Build history of the part. All positions in model axes, mm. Face numbers are marked on the shaded views. A direction names the side the tool comes from. Give positions to 0.01 mm unless a question says otherwise; leave off trailing zeros. Order: outer loops, then holes, each group sorted by start corner. A loop starts at its lowest first (then second) coordinate and runs counter-clockwise, first axis right, second up. Notation, with made-up numbers: (65, 81) - (86, 81) arc R16 cw to (86, 100) - close; hole circle Ø10 at (22, 82.5). An arc over 180 degrees is marked (long way). Answer in a Markdown table with one row per item.
```python
from build123d import *

# Parameters (mm, degrees)
SPUR_START          = 60.68508869
SPUR_GEAR_AI_DEPTH  = 13.97
SKETCH1_R           = 8.73125
BOSS_EXTRUDE1_DEPTH = 0.381
BOSS_EXTRUDE2_START = 0.381
SKETCH2_R           = 8.73125
BOSS_EXTRUDE2_DEPTH = 0.381


# Read off the part's stored shape, not the designer's step: spur gear_ai
with BuildPart() as part:
    # spur gear_ai outline → spur gear_ai (new body)
    with BuildSketch(Plane.YZ.offset(SPUR_START)):
        with BuildLine():
            ThreePointArc((-11.323917399, -24.217086363), (-11.097675416, -23.865456059), (-10.883753605, -23.506197427))
            ThreePointArc((-10.883753605, -23.506197427), (-11.804950291, -22.339121223), (-13.067398654, -21.553695012))
            ThreePointArc((-13.067398654, -21.553695012), (-12.757964709, -20.844772424), (-12.509041094, -20.112408009))
            ThreePointArc((-12.509041094, -20.112408009), (-11.04694228, -20.382476998), (-9.57991556, -20.14060347))
            ThreePointArc((-9.57991556, -20.14060347), (-9.495974711, -19.730989946), (-9.42627775, -19.318713778))
            ThreePointArc((-9.42627775, -19.318713778), (-10.70686463, -18.563222253), (-12.167791342, -18.286883074))
            ThreePointArc((-12.167791342, -18.286883074), (-12.135345159, -17.514052013), (-12.167791342, -16.741220953))
            ThreePointArc((-12.167791342, -16.741220953), (-10.70686463, -16.464881774), (-9.42627775, -15.709390249))
            ThreePointArc((-9.42627775, -15.709390249), (-9.495974711, -15.297114081), (-9.57991556, -14.887500557))
            ThreePointArc((-9.57991556, -14.887500557), (-11.04694228, -14.645627029), (-12.509041094, -14.915696018))
            ThreePointArc((-12.509041094, -14.915696018), (-12.757964709, -14.183331603), (-13.067398654, -13.474409015))
            ThreePointArc((-13.067398654, -13.474409015), (-11.804950291, -12.688982804), (-10.883753605, -11.5219066))
            ThreePointArc((-10.883753605, -11.5219066), (-11.097675416, -11.162647968), (-11.323917399, -10.811017664))
            ThreePointArc((-11.323917399, -10.811017664), (-12.779253872, -11.115428493), (-14.045060241, -11.895431337))
            ThreePointArc((-14.045060241, -11.895431337), (-14.54173514, -11.302443439), (-15.086366078, -10.753173247))
            ThreePointArc((-15.086366078, -10.753173247), (-14.192896711, -9.564736168), (-13.755502936, -8.143695392))
            ThreePointArc((-13.755502936, -8.143695392), (-14.084758271, -7.885974166), (-14.422746154, -7.639816704))
            ThreePointArc((-14.422746154, -7.639816704), (-15.669841124, -8.44939952), (-16.568400884, -9.633992513))
            ThreePointArc((-16.568400884, -9.633992513), (-17.245748371, -9.260467435), (-17.952020875, -8.945031621))
            ThreePointArc((-17.952020875, -8.945031621), (-17.548198493, -7.514088685), (-17.653680083, -6.031002769))
            ThreePointArc((-17.653680083, -6.031002769), (-18.053801184, -5.909625629), (-18.45788783, -5.802185936))
            ThreePointArc((-18.45788783, -5.802185936), (-19.328314212, -7.007602095), (-19.738271888, -8.436799389))
            ThreePointArc((-19.738271888, -8.436799389), (-20.504812431, -8.333183761), (-21.277340486, -8.294183681))
            ThreePointArc((-21.277340486, -8.294183681), (-21.41770354, -6.813991662), (-22.051814621, -5.469159576))
            ThreePointArc((-22.051814621, -5.469159576), (-22.468762916, -5.500519177), (-22.884374185, -5.546307581))
            ThreePointArc((-22.884374185, -5.546307581), (-23.260576072, -6.98475895), (-23.126564609, -8.465539531))
            ThreePointArc((-23.126564609, -8.465539531), (-23.87877266, -8.645827218), (-24.613222072, -8.888530048))
            ThreePointArc((-24.613222072, -8.888530048), (-25.278813753, -7.55899708), (-26.355914109, -6.53404585))
            ThreePointArc((-26.355914109, -6.53404585), (-26.733378421, -6.713906903), (-27.104383709, -6.906739426))
            ThreePointArc((-27.104383709, -6.906739426), (-26.935552952, -8.383955178), (-26.275671339, -9.716331423))
            ThreePointArc((-26.275671339, -9.716331423), (-26.911957033, -10.156173575), (-27.509136339, -10.647800953))
            ThreePointArc((-27.509136339, -10.647800953), (-28.610064803, -9.648487829), (-29.984686063, -9.081842798))
            ThreePointArc((-29.984686063, -9.081842798), (-30.271687745, -9.385914073), (-30.547980731, -9.699747614))
            ThreePointArc((-30.547980731, -9.699747614), (-29.856918859, -11.016221575), (-28.760287766, -12.020248689))
            ThreePointArc((-28.760287766, -12.020248689), (-29.194717194, -12.660242185), (-29.573974019, -13.33439711))
            ThreePointArc((-29.573974019, -13.33439711), (-30.961552776, -12.800266607), (-32.448044722, -12.768456326))
            ThreePointArc((-32.448044722, -12.768456326), (-32.605822607, -13.155671311), (-32.750088392, -13.548120911))
            ThreePointArc((-32.750088392, -13.548120911), (-31.63012714, -14.526055979), (-30.244852672, -15.066134537))
            ThreePointArc((-30.244852672, -15.066134537), (-30.418753733, -15.819844709), (-30.528867342, -16.585478823))
            ThreePointArc((-30.528867342, -16.585478823), (-32.015696192, -16.588668223), (-33.41329985, -17.095988847))
            ThreePointArc((-33.41329985, -17.095988847), (-33.420545159, -17.514052013), (-33.41329985, -17.93211518))
            ThreePointArc((-33.41329985, -17.93211518), (-32.015696192, -18.439435804), (-30.528867342, -18.442625204))
            ThreePointArc((-30.528867342, -18.442625204), (-30.418753733, -19.208259318), (-30.244852672, -19.96196949))
            ThreePointArc((-30.244852672, -19.96196949), (-31.63012714, -20.502048048), (-32.750088392, -21.479983116))
            ThreePointArc((-32.750088392, -21.479983116), (-32.605822607, -21.872432716), (-32.448044722, -22.259647701))
            ThreePointArc((-32.448044722, -22.259647701), (-30.961552776, -22.22783742), (-29.573974019, -21.693706917))
            ThreePointArc((-29.573974019, -21.693706917), (-29.194717194, -22.367861842), (-28.760287766, -23.007855338))
            ThreePointArc((-28.760287766, -23.007855338), (-29.856918859, -24.011882452), (-30.547980731, -25.328356413))
            ThreePointArc((-30.547980731, -25.328356413), (-30.271687745, -25.642189954), (-29.984686063, -25.946261229))
            ThreePointArc((-29.984686063, -25.946261229), (-28.610064803, -25.379616198), (-27.509136339, -24.380303074))
            ThreePointArc((-27.509136339, -24.380303074), (-26.911957033, -24.871930452), (-26.275671339, -25.311772604))
            ThreePointArc((-26.275671339, -25.311772604), (-26.935552952, -26.644148849), (-27.104383709, -28.121364601))
            ThreePointArc((-27.104383709, -28.121364601), (-26.733378421, -28.314197124), (-26.355914109, -28.494058177))
            ThreePointArc((-26.355914109, -28.494058177), (-25.278813753, -27.469106947), (-24.613222072, -26.139573979))
            ThreePointArc((-24.613222072, -26.139573979), (-23.87877266, -26.382276809), (-23.126564609, -26.562564496))
            ThreePointArc((-23.126564609, -26.562564496), (-23.260576072, -28.043345077), (-22.884374185, -29.481796446))
            ThreePointArc((-22.884374185, -29.481796446), (-22.468762916, -29.527584851), (-22.051814621, -29.558944451))
            ThreePointArc((-22.051814621, -29.558944451), (-21.41770354, -28.214112365), (-21.277340486, -26.733920346))
            ThreePointArc((-21.277340486, -26.733920346), (-20.504812431, -26.694920266), (-19.738271888, -26.591304638))
            ThreePointArc((-19.738271888, -26.591304638), (-19.328314212, -28.020501932), (-18.45788783, -29.225918091))
            ThreePointArc((-18.45788783, -29.225918091), (-18.053801184, -29.118478398), (-17.653680083, -28.997101258))
            ThreePointArc((-17.653680083, -28.997101258), (-17.548198493, -27.514015342), (-17.952020875, -26.083072406))
            ThreePointArc((-17.952020875, -26.083072406), (-17.245748371, -25.767636592), (-16.568400884, -25.394111514))
            ThreePointArc((-16.568400884, -25.394111514), (-15.669841124, -26.578704507), (-14.422746154, -27.388287323))
            ThreePointArc((-14.422746154, -27.388287323), (-14.084758271, -27.142129861), (-13.755502936, -26.884408635))
            ThreePointArc((-13.755502936, -26.884408635), (-14.192896711, -25.463367859), (-15.086366078, -24.27493078))
            ThreePointArc((-15.086366078, -24.27493078), (-14.54173514, -23.725660588), (-14.045060241, -23.13267269))
            ThreePointArc((-14.045060241, -23.13267269), (-12.779253872, -23.912675534), (-11.323917399, -24.217086363))
        make_face()
        with BuildLine():
            Line((-13.481545159, -19.101552014), (-15.207184097, -19.101552014))
            ThreePointArc((-15.207184097, -19.101552014), (-27.705545159, -17.514052014), (-15.207184097, -15.926552014))
            Line((-15.207184097, -15.926552014), (-13.481545159, -15.926552014))
            Line((-13.481545159, -15.926552014), (-13.481545159, -19.101552014))
        make_face(mode=Mode.SUBTRACT)
    extrude(amount=SPUR_GEAR_AI_DEPTH)

    # Sketch1 → Boss-Extrude1 (add)
    with BuildSketch(Plane(origin=(74.65508869, 0, 0), x_dir=(0, 0, -1), z_dir=(1, 0, 0))):
        with Locations(Location((17.514052014, -21.355545159, 0), (0, 0, 180))):
            Circle(SKETCH1_R)
        with BuildLine():
            Line((15.926552014, -13.481545159), (15.926552014, -15.207184097))
            ThreePointArc((15.926552014, -15.207184097), (17.514052014, -27.705545159), (19.101552014, -15.207184097))
            Line((19.101552014, -15.207184097), (19.101552014, -13.481545159))
            Line((19.101552014, -13.481545159), (15.926552014, -13.481545159))
        make_face(mode=Mode.SUBTRACT)
    extrude(amount=BOSS_EXTRUDE1_DEPTH)

    # Sketch2 → Boss-Extrude2 (add)
    with BuildSketch(Plane.ZY.offset(-60.68508869).offset(BOSS_EXTRUDE2_START)):
        with Locations((-17.514052014, -21.355545159)):
            Circle(SKETCH2_R)
        with BuildLine():
            Line((-19.101552014, -13.481545159), (-19.101552014, -15.207184097))
            ThreePointArc((-19.101552014, -15.207184097), (-17.514052014, -27.705545159), (-15.926552014, -15.207184097))
            Line((-15.926552014, -15.207184097), (-15.926552014, -13.481545159))
            Line((-15.926552014, -13.481545159), (-19.101552014, -13.481545159))
        make_face(mode=Mode.SUBTRACT)
    extrude(amount=-BOSS_EXTRUDE2_DEPTH)


solid = part.part
```
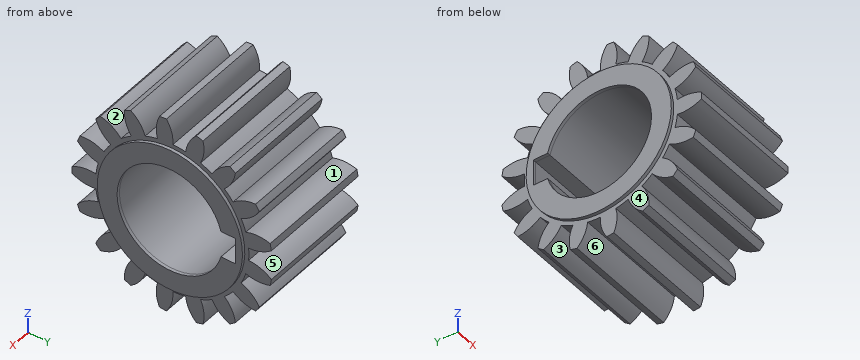
1. Which spindle directions (+Z, -Z, +X, -X, +Y, -Y) get a long thin tool onto all of the face, cutting with end or side? Do the marked faces 1, 2 and 3. Say none if no direction does.
Check result:
| item | result |
|---|---|
| face 1 | +X, -X |
| face 2 | +Z, +X, -X |
| face 3 | -Z, +X, -X |
2. Two-plate mould, pull along Z, no slides. Class the marked faces 4, 5 and 6: +Z half, -Z half, draft (parallel to the pull), parting line (faces both ways), or undercut.
Check result:
| item | result |
|---|---|
| face 4 | draft |
| face 5 | undercut |
| face 6 | -Z half |
3. Drop flat-ended pins along their axis: P1, Ø6, axis at x = 62, z = -23.5, coming from the +Y side; P2, Ø2, axis at y = -15, z = -25, coming from the +X side; P3, Ø12, axis at y = -18, z = -20, coming from the +X side; P4, Ø0.9, axis at x = 70, y = -14.5, coming from the +Z side. Give the stop position or say it passes through.
Check result:
| item | result |
|---|---|
| P1 | stops at y = -10.88 |
| P2 | stops at x = 74.66 |
| P3 | stops at x = 75.04 |
| P4 | stops at z = -7.64 |
4. Cut at A-A on y = -25.5. Write the cut outline in (x, z), and give its area (3 significant figures).
Check result:
| item | result |
|---|---|
| outline | (60.3, -25.2) - (60.69, -25.2) - (60.69, -27.74) - (74.66, -27.74) - (74.66, -25.2) - (75.04, -25.2) - (75.04, -22.33) - (60.3, -22.33) - close; (60.3, -12.7) - (75.04, -12.7) - (75.04, -9.83) - (74.66, -9.83) - (74.66, -7.28) - (60.69, -7.28) - (60.69, -9.83) - (60.3, -9.83) - close |
| area | 156 mm² |
5. Cut at B-B on z = -10.25. Write the cut outline in (x, y), and give its area (3 significant figures).
Check result:
| item | result |
|---|---|
| outline | (60.3, -26.2) - (60.69, -26.2) - (60.69, -27.03) - (74.66, -27.03) - (74.66, -26.2) - (75.04, -26.2) - (75.04, -16.51) - (74.66, -16.51) - (74.66, -14.63) - (60.69, -14.63) - (60.69, -16.51) - (60.3, -16.51) - close; (60.69, -30.33) - (74.66, -30.33) - (74.66, -27.86) - (60.69, -27.86) - close |
| area | 215 mm² |
6. Probe line 1 (Z direction, x = 71.25, y = -13); line 2 (Z direction, x = 73, y = -15.5); line 3 (Z direction, x = 70.25, y = -29). List the from-to ranges inside material, lowest first.
Check result:
| item | result |
|---|---|
| line 1 | z = -23.82 to -21.58, -21.41 to -13.62, -13.45 to -11.21 |
| line 2 | z = -26.73 to -19.97, -15.06 to -8.3 |
| line 3 | z = -25.6 to -23.17, -22.67 to -12.36, -11.86 to -9.43 |
